Job drawing, mm, ordinate dimensions from the low corner. One solid piece. Give positions to 0.01 mm unless a question says otherwise; leave off trailing zeros. Loops run counter-clockwise (first coordinate to the right, second up) from the corner with the lowest first, then second, coordinate; pieces in that order, holes last. Notation, with made-up numbers: (-34, -14) -> (6, -14) arc R27 ccw to (6, 25) -> close; hole circle Ø7 at (-22, 6.5). An arc over 180 degrees is marked (long way). Answer as a JSON object with one key per item and string values. Group by question number.
Q1. Band-saw the part on D-D, the plane y = 14. Write the cut outline in (x, z), plus the area to 3 significant figures.
Q2. Band-saw the part on A-A, the plane y = 35. Write the cut outline in (x, z).
Q3. Band-saw the part on C-C, the plane x = 0.45. Count the separate pieces of the cut face and the enclosed holes in it, plus the area to 3 significant figures.
Q4. Drop a flat-ended pin along its axis: pin 1 (4 mm diameter, centred on y = 25, z = 10, fed in from -X). Give the stop position or say it passes through.
Q5. Wall check: probe 1 along Y at (x, z) = (2.25, 10); probe 2 along Y at (x, z) = (1.8, 5); probe 3 along Z at (x, y) = (1.75, 60). Give the ranges that are in metal, low to high. Write a range as from..to.
Q6. Band-saw the part on B-B, the plane z = 15. Write the cut outline in (x, y).
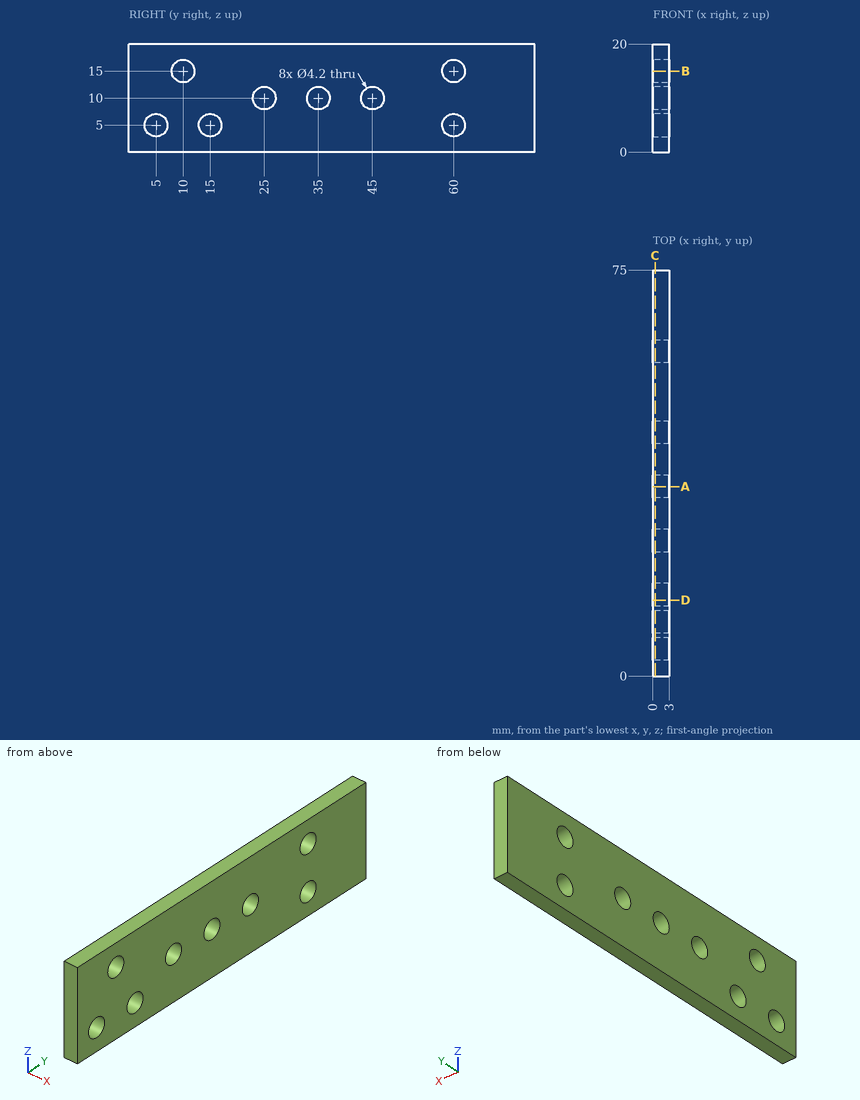
Worked answers:
{
 "1": {"outline": "(0, 0) -> (3, 0) -> (3, 3.15) -> (0, 3.15) -> close; (0, 6.85) -> (3, 6.85) -> (3, 20) -> (0, 20) -> close", "area": "48.9 mm2"},
 "2": {"outline": "(0, 0) -> (3, 0) -> (3, 7.9) -> (0, 7.9) -> close; (0, 12.1) -> (3, 12.1) -> (3, 20) -> (0, 20) -> close"},
 "3": {"separate pieces": "1", "enclosed holes": "8", "area": "1,390 mm2"},
 "4": {"pin 1": "through"},
 "5": {"probe 1": "0..22.9, 27.1..32.9, 37.1..42.9, 47.1..75", "probe 2": "0..2.9, 7.1..12.9, 17.1..57.9, 62.1..75", "probe 3": "0..2.9, 7.1..12.9, 17.1..20"},
 "6": {"outline": "(0, 0) -> (3, 0) -> (3, 7.9) -> (0, 7.9) -> close; (0, 12.1) -> (3, 12.1) -> (3, 57.9) -> (0, 57.9) -> close; (0, 62.1) -> (3, 62.1) -> (3, 75) -> (0, 75) -> close"}
}
